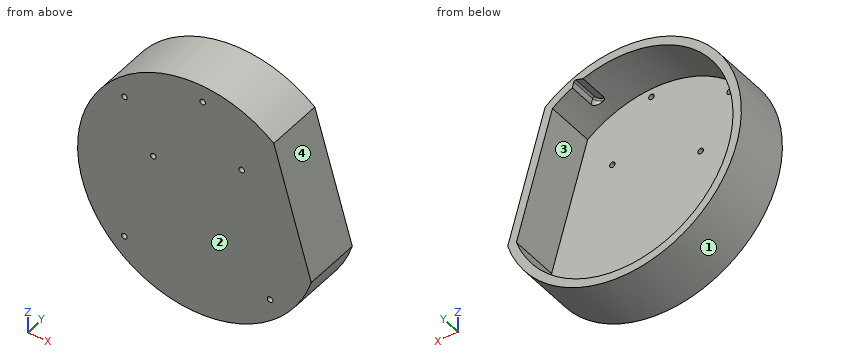
```python
from build123d import *

# Parameters (mm, degrees)
BOSS_EXTRUDE1_DEPTH = 5
SKETCH2_R           = 1.65
CUT_EXTRUDE1_DEPTH  = 6
BOSS_EXTRUDE3_DEPTH = 30
CUT_EXTRUDE2_DEPTH  = 15
FILLET1_R           = 1
SKETCH5_R           = 1.65
CUT_EXTRUDE3_DEPTH  = 6


with BuildPart() as part:
    # Sketch1 → Boss-Extrude1 (new body)
    with BuildSketch(Plane(origin=(0, 0, 0), x_dir=(1, 0, 0), z_dir=(0, 1, 0))):
        with BuildLine():
            Line((45.736375855, -55.017005995), (68.149505263, 21.779163377))
            ThreePointArc((68.149505263, 21.779163377), (-68.679774221, 20.044341793), (45.736375855, -55.017005995))
        make_face()
    extrude(amount=BOSS_EXTRUDE1_DEPTH)

    # Sketch2 → Cut-Extrude1 (cut, through all)
    with BuildSketch(Plane(origin=(0, 5, 0), x_dir=(1, 0, 0), z_dir=(0, 1, 0))):
        with Locations((43.522422382, 43.522422382)):
            Circle(SKETCH2_R)
        with Locations((-43.522422382, -43.522422382)):
            Circle(SKETCH2_R)
        with Locations((-43.522422382, 43.522422382)):
            Circle(SKETCH2_R)
        with Locations((3.221278107, -61.465647864)):
            Circle(SKETCH2_R)
    extrude(amount=-CUT_EXTRUDE1_DEPTH, mode=Mode.SUBTRACT)

    # Sketch3 → Boss-Extrude3 (add)
    with BuildSketch(Plane(origin=(0, 5, 0), x_dir=(1, 0, 0), z_dir=(0, 1, 0))):
        with BuildLine():
            Line((45.736375855, -55.017005995), (68.149505263, 21.779163377))
            ThreePointArc((68.149505263, 21.779163377), (-68.679774221, 20.044341793), (45.736375855, -55.017005995))
        make_face()
        with BuildLine():
            Line((41.373300987, -52.119928918), (62.91305896, 21.683727477))
            ThreePointArc((62.91305896, 21.683727477), (-63.880013635, 18.643521205), (41.373300987, -52.119928918))
        make_face(mode=Mode.SUBTRACT)
    extrude(amount=BOSS_EXTRUDE3_DEPTH)

    # Sketch4 → Cut-Extrude2 (cut)
    with BuildSketch(Plane(origin=(-10.769878987, 0, 36.901828197), x_dir=(0, -1, 0), z_dir=(0.280164118, 0, -0.959952117))):
        with BuildLine():
            Line((-19, -45.06852177), (-35, -45.06852177))
            ThreePointArc((-35, -45.06852177), (-38.5, -41.56852177), (-35, -38.06852177))
            Line((-35, -38.06852177), (-19, -38.06852177))
            ThreePointArc((-19, -38.06852177), (-15.5, -41.56852177), (-19, -45.06852177))
        make_face()
    extrude(amount=-CUT_EXTRUDE2_DEPTH, mode=Mode.SUBTRACT)

    # Fillet1
    fillet1_edges = [part.edges().sort_by_distance(p)[0] for p in [
        (26.529321315, 15.921147738, 63.413460481),
        (28.291282139, 27, 63.927692588),
    ]]
    fillet(fillet1_edges, radius=FILLET1_R)

    # Sketch5 → Cut-Extrude3 (cut, through all)
    with BuildSketch(Plane(origin=(0, 5, 0), x_dir=(1, 0, 0), z_dir=(0, 1, 0))):
        with Locations((26.569138232, -29.673397669)):
            Circle(SKETCH5_R)
        with Locations((-26.228228211, -14.264371202)):
            Circle(SKETCH5_R)
    extrude(amount=-CUT_EXTRUDE3_DEPTH, mode=Mode.SUBTRACT)


solid = part.part
```
Geometry check sheet. Reference: the model listing, model coordinates, mm. Face numbers are marked on the shaded views. Round coordinates to 2 decimals unless told otherwise and drop trailing zeros. Order: outer loops, then holes, each group sorted by start corner. A loop starts at its lowest first (then second) coordinate and runs counter-clockwise, first axis right, second up. Notation, with made-up numbers: (38.25, 29) -> (89.25, 29) arc R20 ccw to (89.25, 49) -> close; hole circle Ø3 at (53.5, -1.5). An arc over 180 degrees is marked (long way). Return JSON: item names as keys, results as strings. Group by question number.
Q1. Section check A-A, the plane y = 30.5. Record the boundary of the cut face in (x, z) (1 decimal).
Q2. Section check C-C, the plane y = 2.5. Count the separate pieces of the cut face and the enclosed holes in it, plus the area to 3 significant figures.
Q3. Release check for a two-part mould opening along Z. For the marked faces 1, 2, 3 and 4 record: released by +Z, released by -Z, zero draft, split by the parting line, or undercut.
Q4. Gauge pin test, flat ends, axial feed: pin 1 (2 mm diameter, centred on x = -56, y = 3.5, fed in from +Z); pin 2 (1 mm diameter, centred on x = 4.5, z = 16, fed in from +Y); pin 3 (1.5 mm diameter, centred on y = 28.5, z = -18, fed in from +X); pin 4 (2 mm diameter, centred on x = -43.52, z = 43.52, fed in from -Y). Record the tip position at first contact, or that the pin passes through.
Q5. Material ranges on probe 1 along Z at (x, y) = (0, 25) (3 decimals); probe 2 along Y at (x, z) = (36.5, 8); probe 3 along Z at (x, y) = (29, 11.5), recorded low to high. Write a range as from..to.
Q6. Section check B-B, the plane x = 14.5. Record the boundary of the cut face in (y, z), plus the area to 3 significant figures.
Q7. Section check D-D, the plane z = 0. Record the boundary of the cut face in (x, y) (3 decimals), plus the area to 3 significant figures.
Numbers:
{
 "1": {"outline": "(45.7, 55) arc R71.5 ccw (long way) to (68.1, -21.8) -> close; hole (23.1, 62.4) arc R66.5 ccw (long way) to (62.9, -21.7) -> (41.4, 52.1) arc R66.5 ccw to (29.5, 59.6) -> (28.6, 63) arc R1 ccw to (27.3, 63.6) -> close"},
 "2": {"separate pieces": "1", "enclosed holes": "6", "area": "15,400 mm^2"},
 "3": {"face 1": "split by the parting line", "face 2": "zero draft", "face 3": "undercut", "face 4": "released by +Z"},
 "4": {"pin 1": "z = 45.76", "pin 2": "y = 5", "pin 3": "x = 67.27", "pin 4": "through"},
 "5": {"probe 1": "-71.545..-66.545, 66.545..71.545", "probe 2": "0..5", "probe 3": "-65.4..-59.89, 59.89..65.4"},
 "6": {"outline": "(0, -70.06) -> (35, -70.06) -> (35, -64.95) -> (5, -64.95) -> (5, 64.95) -> (35, 64.95) -> (35, 70.06) -> (0, 70.06) -> close", "area": "1,010 mm^2"},
 "7": {"outline": "(-71.545, 0) -> (61.793, 0) -> (61.793, 35) -> (56.585, 35) -> (56.585, 5) -> (-66.545, 5) -> (-66.545, 35) -> (-71.545, 35) -> close", "area": "973 mm^2"}
}
